The model under review builds one solid part; all positions refer to its coordinate system, in mm. A direction names the side the tool comes from. Round coordinates to 2 decimals unless told otherwise and drop trailing zeros. Order: outer loops, then holes, each group sorted by start corner. A loop starts at its lowest first (then second) coordinate and runs counter-clockwise, first axis right, second up. Notation, with made-up numbers: M 82.25,-7 L 87.25,-7 A22 cw 87.25,31 Z; hole C 74,5.5 d3. An arc over 180 degrees is marked long. Answer as a JSON object with one key per item and string values. Group by question number.
1. To check wall thickness, follow probe 1 along Y at (x, z) = (0, 13.5) (3 decimals); probe 2 along Z at (x, y) = (2.5, 2); probe 3 along Z at (x, y) = (-5, 0.5). State the ranges of each line that lie inside material, in increasing order. Write a range as [from, to].
2. Add section A-A on x = 0. State the section outline as (y, z) points (1 decimal).
3. Mouldability with a two-part tool opening along X and no side actions: class faces 1 (the face through (5.45, 1.72, 12.45)), 2 (the face through (1.588, 0, 4)), 3 (the face through (0, 0, 10.287)) as released by +X, released by -X, zero draft, split by the parting line, or undercut.
4. Add section C-C on z = 6.5. State the section outline as (x, y) points, and give its area (3 significant figures).
5. Machinability: for faces 4 (the face through (-3.83, -2.937, 13.506)), 5 (the face through (0, -1.588, 4)), 6 (the face through (-1.588, 0, 4)), 7 (the face through (0, 1.588, 4)), which of the approach directions +Z, -Z, +X, -X, +Y, -Y give a long, thin tool a straight path to every point of the face, cutting with its end or side? Answer none if there is none.
6. Add section D-D on z = 11.25. State the section outline as (x, y) points (3 decimals).
7. Clearance check with flat-ended pins moving along their axes: P1, Ø4, axis at y = -3.5, z = 7.5, coming from the -X side; P2, Ø1.6, axis at y = 0, z = 4.5, coming from the +X side; P3, Ø1.5, axis at y = -2.5, z = 7.5, coming from the +X side; P4, Ø3.5, axis at x = 0, z = 4, coming from the -Y side. State where each tip first meets the part, or that it passes through.
```python
from build123d import *

# Parameters (mm, degrees)
F1_DEPTH = 8.382
F2_R     = 5.715
F3_DEPTH = 8.255
F4_R     = 4.826
F5_DEPTH = 6.35


with BuildPart() as f1:
    # F0 (on Top) → F1 (new body)
    with BuildSketch(Plane.XY):
        Polygon((1.5875, -1.5875), (1.5875, 0), (1.5875, 1.5875), (-1.5875, 1.5875), (-1.5875, -1.5875), align=None)
    extrude(amount=F1_DEPTH)

    # F2 (on face) → F3 (join)
    with BuildSketch(Plane.XY.offset(8.382)):
        Circle(F2_R)
    extrude(amount=F3_DEPTH)

    # F4 (on face) → F5 (cut)
    with BuildSketch(Plane.XY.offset(16.637)):
        Circle(F4_R)
    extrude(amount=-F5_DEPTH, mode=Mode.SUBTRACT)


solid = f1.part
```
Recorded:
{
 "1": {"probe 1": "y = [-5.715, -4.826], [4.826, 5.715]", "probe 2": "z = [8.38, 10.29]", "probe 3": "z = [8.38, 16.64]"},
 "2": {"outline": "M -5.7,8.4 L -1.6,8.4 L -1.6,0 L 1.6,0 L 1.6,8.4 L 5.7,8.4 L 5.7,16.6 L 4.8,16.6 L 4.8,10.3 L -4.8,10.3 L -4.8,16.6 L -5.7,16.6 Z"},
 "3": {"face 1": "split by the parting line", "face 2": "released by +X", "face 3": "undercut"},
 "4": {"outline": "M -1.59,-1.59 L 1.59,-1.59 L 1.59,1.59 L -1.59,1.59 Z", "area": "10.1 mm²"},
 "5": {"face 4": "+Z", "face 5": "-Z, +X, -X, -Y", "face 6": "-Z, -X, +Y, -Y", "face 7": "-Z, +X, -X, +Y"},
 "6": {"outline": "C 0,0 d11.43; hole C 0,0 d9.652"},
 "7": {"P1": "stops at x = -5.45", "P2": "stops at x = 1.59", "P3": "passes through", "P4": "stops at y = -1.59"}
}
